Work out the finished part from the listing and answer in its coordinate system (mm). Give positions to 0.01 mm unless a question says otherwise; leave off trailing zeros. Order: outer loops, then holes, each group sorted by start corner. A loop starts at its lowest first (then second) coordinate and runs counter-clockwise, first axis right, second up.
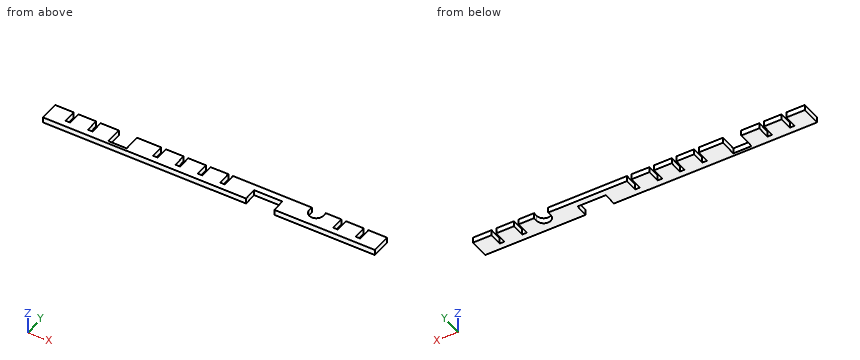
Autodesk Inventor part; units mm, degrees
ref_plane "YZ Plane" through (0, 0, 0) normal (1, 0, 0) x (0, 1, 0)
ref_plane "XZ Plane" through (0, 0, 0) normal (0, 1, 0) x (-1, 0, 0)
ref_plane "XY Plane" through (0, 0, 0) normal (0, 0, 1) x (1, 0, 0)
sketch "Sketch1" plane through (0, 0, 0) normal (0, 0, 1) x (1, 0, 0)
  line L0 (89.1, -5.2) -> (-89.1, -5.2)
  line L1 (-89.1, -5.2) -> (-89.1, 5.2)
  line L2 (-89.1, 5.2) -> (89.1, 5.2)
  line L3 (89.1, 5.2) -> (89.1, -5.2)
  line L4 (89.1, -5.2) -> (-89.1, 5.2) construction
  line L5 (-89.1, -5.2) -> (89.1, 5.2) construction
  point P0 (0, 0)
  dimension "d0" = 10.4
  dimension "d1" = 178.2
extrude "Extrusion1" add sketch "Sketch1" along normal blind 3
sketch "Sketch2" plane through (0, 0, 0) normal (0, 0, -1) x (-1, 0, 0)
  line L0 (-89.1, -5.2) -> (89.1, -5.2)
  line L1 (45.1, 5.2) -> (54.9, 5.2)
  line L2 (54.9, 5.2) -> (54.9, -3.7)
  line L3 (54.9, -3.7) -> (45.1, -3.7)
  line L4 (45.1, -3.7) -> (45.1, 5.2)
  line L5 (89.1, 5.2) -> (-89.1, 5.2)
  arc A0 (-56.275, 3) -> (-48.725, 3) centre (-52.5, 3) ccw
  line L6 (-56.275, 3) -> (-56.275, 5.2)
  line L7 (-48.725, 3) -> (-48.725, 5.2)
  line L8 (-56.275, 5.2) -> (-48.725, 5.2)
  arc A1 (-48.725, 3) -> (-56.275, 3) centre (-52.5, 3) ccw construction
  line L9 (-35.1, 1.8) -> (-19.9, 1.8)
  line L10 (-19.9, 1.8) -> (-19.9, -5.2)
  line L11 (-19.9, -5.2) -> (-35.1, -5.2)
  line L12 (-35.1, -5.2) -> (-35.1, 1.8)
  line L13 (89.1, -5.2) -> (-89.1, -5.2)
  point P0 (0, 0)
  point P1 (50, 2.9)
  point P2 (50, 5.2)
  point P3 (-27.5, -2.25)
  point P4 (-27.5, 1.8)
  dimension "d4" = 50
  dimension "d5" = 8.1
  dimension "d6" = 1.5
  dimension "d7" = 9.8
  dimension "d8" = 52.5
  dimension "d9" = 7.55
  dimension "d10" = 8.2
  dimension "d13" = 27.5
  dimension "d14" = 2.95
  dimension "d16" = 7
  dimension "d17" = 15.2
extrude "Extrusion2" cut sketch "Sketch2" against normal through all
sketch "Sketch3" plane through (0, 0, 0) normal (0, 0, -1) x (-1, 0, 0)
  line L0 (-56.275, 5.2) -> (-89.1, 5.2)
  line L1 (45.1, 5.2) -> (-48.725, 5.2)
  line L2 (89.1, 5.2) -> (54.9, 5.2)
  line L3 (-79.1, 5.2) -> (-76.6, 5.2)
  line L4 (-76.6, 5.2) -> (-76.6, -1.8)
  line L5 (-76.6, -1.8) -> (-79.1, -1.8)
  line L6 (-79.1, -1.8) -> (-79.1, 5.2)
  line L7 (-67.1, 5.2) -> (-64.6, 5.2)
  line L8 (-64.6, 5.2) -> (-64.6, -1.8)
  line L9 (-64.6, -1.8) -> (-67.1, -1.8)
  line L10 (-67.1, -1.8) -> (-67.1, 5.2)
  line L11 (-89.1, 5.2) -> (-89.1, -5.2)
  line L12 (64.6, 5.2) -> (67.1, 5.2)
  line L13 (67.1, 5.2) -> (67.1, -1.8)
  line L14 (67.1, -1.8) -> (64.6, -1.8)
  line L15 (64.6, -1.8) -> (64.6, 5.2)
  line L16 (76.6, 5.2) -> (79.1, 5.2)
  line L17 (79.1, 5.2) -> (79.1, -1.8)
  line L18 (79.1, -1.8) -> (76.6, -1.8)
  line L19 (76.6, -1.8) -> (76.6, 5.2)
  line L20 (89.1, -5.2) -> (89.1, 5.2)
  line L21 (32.1, 5.2) -> (29.6, 5.2)
  line L22 (29.6, 5.2) -> (29.6, -1.8)
  line L23 (29.6, -1.8) -> (32.1, -1.8)
  line L24 (32.1, -1.8) -> (32.1, 5.2)
  line L25 (20.1, 5.2) -> (17.6, 5.2)
  line L26 (17.6, 5.2) -> (17.6, -1.8)
  line L27 (17.6, -1.8) -> (20.1, -1.8)
  line L28 (20.1, -1.8) -> (20.1, 5.2)
  line L29 (8.1, 5.2) -> (5.6, 5.2)
  line L30 (5.6, 5.2) -> (5.6, -1.8)
  line L31 (5.6, -1.8) -> (8.1, -1.8)
  line L32 (8.1, -1.8) -> (8.1, 5.2)
  line L33 (-3.9, 5.2) -> (-6.4, 5.2)
  line L34 (-6.4, 5.2) -> (-6.4, -1.8)
  line L35 (-6.4, -1.8) -> (-3.9, -1.8)
  line L36 (-3.9, -1.8) -> (-3.9, 5.2)
  point P0 (0, 0)
  dimension "d18" = 2.5
  dimension "d19" = 10
  dimension "d21" = 7
  dimension "d24" = 12
  dimension "d25" = 10
  dimension "d26" = 12
  dimension "d28" = 12
  dimension "d29" = 12
  dimension "d30" = 35
  dimension "d31" = 12
extrude "Extrusion3" cut sketch "Sketch3" against normal through all
equation "\"d26\" = d24"
equation "\"d28\" = d31"
equation "\"d29\" = d31"
equation "\"d31\" = d24"
properties part number "Back"
1. Straight lines are drawn through the part: probe 1 along X at (y, z) = (-2.75, 0.6); probe 2 along X at (y, z) = (-4, 2); probe 3 along Y at (x, z) = (-19, 0.8). For each, find the intervals that lie inside material, in ascending order.
Findings below:
probe 1: x = -89.1 to -54.9, -45.1 to 19.9, 35.1 to 89.1
probe 2: x = -89.1 to 19.9, 35.1 to 89.1
probe 3: y = -5.2 to -1.8
2. The part is cut by section A-A (x = 52.5). Write down the section's boundary in (y, z) (3 decimals).
Findings below:
outline: (-5.2, 0) - (-0.775, 0) - (-0.775, 3) - (-5.2, 3) - close
3. Given P1, Ø0.8, axis at x = -77.5, z = 1, coming from the +Y side; P2, Ø1.5, axis at x = -48, z = 1, coming from the +Y side, each flat-ended and moving along its own axis, determine where each tip first touches the part or whether it passes through.
Findings below:
P1: stops at y = -1.8
P2: stops at y = -3.7
